from build123d import *

# Parameters (mm, degrees)
SKETCH1_W              = 15
SKETCH1_H              = 7.3
BASE_EXTRUDE1_DEPTH    = 1
NOTCH_W                = 3.06
NOTCH_H                = 2
CUT_EXTRUDE1_DEPTH     = 1
SKETCH5_W              = 4.61
SKETCH5_H              = 1
TOP_LED_EXTRUDE_DEPTH  = 1
SKETCH6_W              = 1
SKETCH6_H              = 1
TOP_CLAMP_DEPTH        = 1
SKETCH7_W              = 1
SKETCH7_H              = 4.61
SIDE_LED_EXTRUDE_DEPTH = 1
SKETCH8_W              = 1
SKETCH8_H              = 1
SIDE_CLAMP_DEPTH       = 1
SKETCH9_R              = 0.375
SCREWHOLES_DEPTH       = 1


with BuildPart() as part:
    # Sketch1 → Base-Extrude1 (new body)
    with BuildSketch(Plane.XY):
        with Locations((1.905405405, 0.163513514)):
            Rectangle(SKETCH1_W, SKETCH1_H)
    extrude(amount=BASE_EXTRUDE1_DEPTH)

    # Notch → Cut-Extrude1 (cut)
    with BuildSketch(Plane(origin=(0, 0, 0), x_dir=(-1, 0, 0), z_dir=(0, 0, -1))):
        with Locations((4.064594595, 2.813513514)):
            Rectangle(NOTCH_W, NOTCH_H)
    extrude(amount=-CUT_EXTRUDE1_DEPTH, mode=Mode.SUBTRACT)

    # Sketch5 → Top-LED-Extrude (add)
    with BuildSketch(Plane.XY.offset(1)):
        with Locations((-0.229594595, 4.313513514)):
            Rectangle(SKETCH5_W, SKETCH5_H)
    extrude(amount=-TOP_LED_EXTRUDE_DEPTH)

    # Sketch6 → Top-Clamp (add)
    with BuildSketch(Plane.XY.offset(1)):
        with Locations((-2.034594595, 4.313513514)):
            Rectangle(SKETCH6_W, SKETCH6_H)
        with Locations((1.575405405, 4.313513514)):
            Rectangle(SKETCH6_W, SKETCH6_H)
    extrude(amount=TOP_CLAMP_DEPTH)

    # Sketch7 → Side-LED-Extrude (add)
    with BuildSketch(Plane.ZY.offset(5.594594595)):
        with Locations((0.5, -0.851486486)):
            Rectangle(SKETCH7_W, SKETCH7_H)
    extrude(amount=SIDE_LED_EXTRUDE_DEPTH)

    # Sketch8 → Side-Clamp (add)
    with BuildSketch(Plane.XY.offset(1)):
        with Locations((-6.094594595, -2.656486486)):
            Rectangle(SKETCH8_W, SKETCH8_H)
        with Locations((-6.094594595, 0.953513514)):
            Rectangle(SKETCH8_W, SKETCH8_H)
    extrude(amount=SIDE_CLAMP_DEPTH)

    # Sketch9 → ScrewHoles (cut)
    with BuildSketch(Plane(origin=(0, 0, 0), x_dir=(-1, 0, 0), z_dir=(0, 0, -1))):
        with Locations((-8.405405405, -0.486486486)):
            Circle(SKETCH9_R)
        with Locations((4.094594595, 1.313513514)):
            Circle(SKETCH9_R)
        with Locations((-1.655405405, -3.486486486)):
            Circle(SKETCH9_R)
    extrude(amount=-SCREWHOLES_DEPTH, mode=Mode.SUBTRACT)


solid = part.part
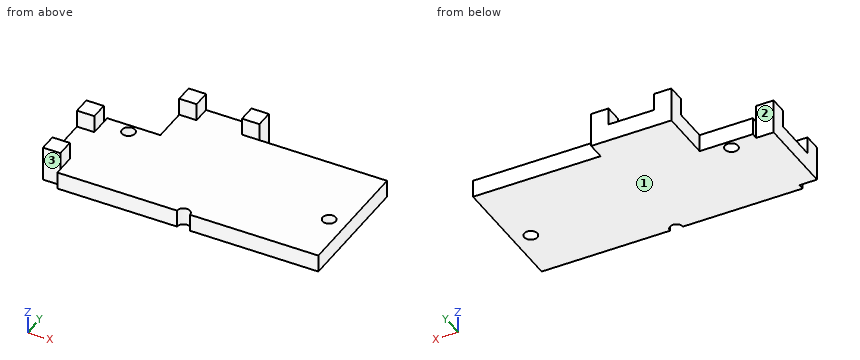
For this review, take the finished solid that the model builds, in its own axes (mm). Face numbers are marked on the shaded views. A direction names the side the tool comes from. Coordinates: 2 decimals unless noted, no trailing zeros. Order: outer loops, then holes, each group sorted by start corner. A loop starts at its lowest first (then second) coordinate and runs counter-clockwise, first axis right, second up. Notation, with made-up numbers: (44.5, -31.5) -> (86.5, -31.5) arc R6 cw to (86.5, -26.5) -> close; hole circle Ø5 at (-39.75, 81). An arc over 180 degrees is marked (long way). Return JSON: item names as keys, results as strings.
1. Machinability: for the marked faces 1, 2 and 3, which of the approach directions +Z, -Z, +X, -X, +Y, -Y give a long, thin tool a straight path to every point of the face, cutting with its end or side? Answer none if there is none.
Answer block:
{"face 1": "-Z, +X, -X, +Y, -Y", "face 2": "+Z, -Z, -X, +Y", "face 3": "+Z, -Z, -X, -Y"}
2. We need section A-A on z = 1.5. Write out the cut boundary in (x, y), and give its area (3 significant figures).
Answer block:
{"outline": "(-6.59, -3.16) -> (-5.59, -3.16) -> (-5.59, -2.16) -> (-6.59, -2.16) -> close; (-6.59, 0.45) -> (-5.59, 0.45) -> (-5.59, 1.45) -> (-6.59, 1.45) -> close; (-2.53, 3.81) -> (-1.53, 3.81) -> (-1.53, 4.81) -> (-2.53, 4.81) -> close; (1.08, 3.81) -> (2.08, 3.81) -> (2.08, 4.81) -> (1.08, 4.81) -> close", "area": "4.00 mm²"}
3. We need section B-B on y = -2.75. Write out the cut boundary in (x, z).
Answer block:
{"outline": "(-6.59, 0) -> (9.41, 0) -> (9.41, 1) -> (-5.59, 1) -> (-5.59, 2) -> (-6.59, 2) -> close"}
4. For pin 1 Ø0.5 at (x, z) = (-6, 1.5) entering from +Y; pin 2 Ø0.8 at (x, z) = (-2, 1.5) entering from -Y; pin 3 Ø0.8 at (y, z) = (4.5, 1.5) entering from +X, all flat-tipped, find the tip position at first contact; note any pin that passes through.
Answer block:
{"pin 1": "y = 1.45", "pin 2": "y = 3.81", "pin 3": "x = 2.08"}
5. For line 1 (Y direction, x = 7.5, z = 0.95); line 2 (Z direction, x = 1.75, y = -2.5); line 3 (X direction, y = -3, z = 1.95), list the stretches that pass through material, from the lowest coordinate up. Write a range as from..to.
Answer block:
{"line 1": "-3.49..3.81", "line 2": "0..1", "line 3": "-6.59..-5.59"}
6. We need section D-D on z = 0.25. Write out the cut boundary in (x, y) (3 decimals), and give its area (3 significant figures).
Answer block:
{"outline": "(-6.595, -3.156) -> (-5.595, -3.156) -> (-5.595, -3.486) -> (1.28, -3.486) arc R0.375 cw to (2.03, -3.486) -> (9.405, -3.486) -> (9.405, 3.814) -> (2.075, 3.814) -> (2.075, 4.814) -> (-2.535, 4.814) -> (-2.535, 1.814) -> (-5.595, 1.814) -> (-5.595, 1.454) -> (-6.595, 1.454) -> close; hole circle Ø0.75 at (-4.095, 1.314); hole circle Ø0.75 at (8.405, -0.486)", "area": "111 mm²"}
7. We need section C-C on x = 1.75. Write out the cut boundary in (y, z).
Answer block:
{"outline": "(-3.12, 0) -> (4.81, 0) -> (4.81, 2) -> (3.81, 2) -> (3.81, 1) -> (-3.12, 1) -> close"}
